Build history of the part. All positions in model axes, mm. A direction names the side the tool comes from. Round coordinates to 2 decimals unless told otherwise and drop trailing zeros. Write each loop counter-clockwise with the first axis right and the second up, starting at its lowest first coordinate (ties: lowest second). Pieces come first, ordered by that corner, then holes. Notation, with made-up numbers: M 50.25,82 L 94.25,82 A23 ccw 94.25,110 Z; hole C -37.5,52 d10. An arc over 180 degrees is marked long. One line per item, written item: value. Start each with the question number.
```python
from build123d import *

# Parameters (mm, degrees)
SKETCH1_W                    = 27.5
SKETCH1_H                    = 23.2
BOSS_EXTRUDE1_REACH          = 62.5
SKETCH2_W                    = 13
SKETCH2_H                    = 10
BOSS_EXTRUDE2_DEPTH          = 16.55326241
BOSS_EXTRUDE3_DEPTH          = 1.5
BOSS_EXTRUDE4_DEPTH          = 1.5
CUT_EXTRUDE1_DEPTH           = 25.05326251
CUT_EXTRUDE2_DEPTH           = 2.5
SKETCH8_R                    = 5.5
BOSS_EXTRUDE5_DEPTH          = 2
SKETCH9_R                    = 2
BOSS_EXTRUDE6_DEPTH          = 8.8
SKETCH10_W                   = 8.8
SKETCH10_H                   = 6
BOSS_EXTRUDE7_DEPTH          = 4.22
CUT_EXTRUDE3_START           = -1
SKETCH11_W                   = 6.8
SKETCH11_H                   = 2.22
CUT_EXTRUDE3_DEPTH           = 5
SKETCH12_R                   = 19.15
BOSS_EXTRUDE8_DEPTH          = 1.5
BOSS_EXTRUDE8_TAPER          = 45
F_7_0_7_DIAMETER_HOLE1_D     = 7
F_7_0_7_DIAMETER_HOLE1_DEPTH = 1.5
SKETCH15_W                   = 1.95
SKETCH15_H                   = 0.1
SKETCH16_W                   = 1.95
SKETCH16_H                   = 0.1
SKETCH17_W                   = 1.95
SKETCH17_H                   = 0.1
SKETCH18_W                   = 1.95
SKETCH18_H                   = 0.1
SKETCH19_W                   = 1.95
SKETCH19_H                   = 0.1
SKETCH20_W                   = 1.95
SKETCH20_H                   = 0.1
SKETCH21_W                   = 2
SKETCH21_H                   = 7
SKETCH22_W                   = 1.95
SKETCH22_H                   = 0.9
SKETCH23_W                   = 1.95
SKETCH23_H                   = 0.9
SKETCH24_W                   = 1.95
SKETCH24_H                   = 0.9
SKETCH25_W                   = 1.95
SKETCH25_H                   = 0.9
SKETCH26_W                   = 1.95
SKETCH26_H                   = 0.9
SKETCH27_W                   = 1.95
SKETCH27_H                   = 0.9


with BuildPart() as part:
    # Sketch1 → Revolve1 (revolve)
    with BuildSketch(Plane.XZ.offset(-27.5)):
        with Locations((41.25, 11.6)):
            Rectangle(SKETCH1_W, SKETCH1_H)
    revolve(axis=Axis((27.5, 27.5, 23.2), (0, 0, -1)))

    # Sketch2 → Boss-Extrude1 (add, up to next)
    with BuildSketch(Plane(origin=(0, 60.5, 0), x_dir=(1, 0, 0), z_dir=(0, 1, 0)), mode=Mode.PRIVATE) as boss_extrude1_sk1:
        with Locations((27.5, -10.7)):
            Rectangle(SKETCH2_W, SKETCH2_H)
    boss_extrude1_tool1 = extrude(boss_extrude1_sk1.sketch, amount=-BOSS_EXTRUDE1_REACH, mode=Mode.PRIVATE) - part.part
    add(boss_extrude1_tool1.solids().sort_by_distance((27.5, 60.5, 10.7))[0])

    # Sketch3 → Boss-Extrude2 (add)
    with BuildSketch(Plane.XY.offset(15.7)):
        with BuildLine():
            Line((34, 60.5), (34, 58))
            add(Edge.make_bspline(
                [(21, 58), (34, 58)],
                knots=[0, 0, 1, 1], degree=1))
            Line((21, 58), (21, 60.5))
            Line((21, 60.5), (34, 60.5))
        make_face()
    extrude(amount=-BOSS_EXTRUDE2_DEPTH)

    # Sketch4 → Boss-Extrude3 (add)
    with BuildSketch(Plane.XY.offset(23.2)):
        with BuildLine():
            Line((64, 32.25), (54.586666462, 32.25))
            ThreePointArc((54.586666462, 32.25), (53.216477037, 17.757679496), (44.640410959, 5.995202578))
            Line((44.640410959, 5.995202578), (66.960616438, 23.785534991))
            ThreePointArc((66.960616438, 23.785534991), (68.483648559, 29.068246028), (64, 32.25))
        make_face()
    extrude(amount=-BOSS_EXTRUDE3_DEPTH)

    # Sketch5 → Boss-Extrude4 (add)
    with BuildSketch(Plane.XY.offset(23.2)):
        with BuildLine():
            Line((-11.960616438, 23.785534991), (10.359589041, 5.995202578))
            ThreePointArc((10.359589041, 5.995202578), (1.783522963, 17.757679496), (0.413333538, 32.25))
            Line((0.413333538, 32.25), (-9, 32.25))
            ThreePointArc((-9, 32.25), (-13.483648559, 29.068246028), (-11.960616438, 23.785534991))
        make_face()
    extrude(amount=-BOSS_EXTRUDE4_DEPTH)

    # Sketch6 → Cut-Extrude1 (cut, through all)
    with BuildSketch(Plane.XY.offset(23.2)):
        with BuildLine():
            Line((63, 25.25), (64, 25.25))
            ThreePointArc((64, 25.25), (66.25, 27.5), (64, 29.75))
            Line((64, 29.75), (63, 29.75))
            ThreePointArc((63, 29.75), (60.75, 27.5), (63, 25.25))
        make_face()
    extrude(amount=-CUT_EXTRUDE1_DEPTH, mode=Mode.SUBTRACT)

    # Sketch7 → Cut-Extrude2 (cut, through all)
    with BuildSketch(Plane(origin=(0, 0, 21.7), x_dir=(-1, 0, 0), z_dir=(0, 0, -1))):
        with BuildLine():
            Line((8, 25.25), (9, 25.25))
            ThreePointArc((9, 25.25), (11.25, 27.5), (9, 29.75))
            Line((9, 29.75), (8, 29.75))
            ThreePointArc((8, 29.75), (5.75, 27.5), (8, 25.25))
        make_face()
    extrude(amount=-CUT_EXTRUDE2_DEPTH, mode=Mode.SUBTRACT)

    # Sketch8 → Boss-Extrude5 (add)
    with BuildSketch(Plane.XY.offset(23.2)):
        with Locations((27.5, 27.5)):
            Circle(SKETCH8_R)
    extrude(amount=BOSS_EXTRUDE5_DEPTH)

    # Sketch9 → Boss-Extrude6 (add)
    with BuildSketch(Plane.XY.offset(25.2)):
        with Locations((27.5, 27.5)):
            Circle(SKETCH9_R)
    extrude(amount=BOSS_EXTRUDE6_DEPTH)

    # Sketch10 → Boss-Extrude7 (add)
    with BuildSketch(Plane(origin=(0, 60.5, 0), x_dir=(-1, 0, 0), z_dir=(0, 1, 0))):
        with Locations((-27.6, 3.14673759)):
            Rectangle(SKETCH10_W, SKETCH10_H)
    extrude(amount=BOSS_EXTRUDE7_DEPTH)

    # Sketch11 → Cut-Extrude3 (cut)
    with BuildSketch(Plane.XY.offset(6.14673759).offset(CUT_EXTRUDE3_START)):
        with Locations((27.6, 62.61)):
            Rectangle(SKETCH11_W, SKETCH11_H)
    extrude(amount=-CUT_EXTRUDE3_DEPTH, mode=Mode.SUBTRACT)

    # Sketch12 → Boss-Extrude8 (add)
    with BuildSketch(Plane(origin=(0, 0, 0), x_dir=(-1, 0, 0), z_dir=(0, 0, -1))):
        with Locations((-27.5, 27.5)):
            Circle(SKETCH12_R)
    extrude(amount=BOSS_EXTRUDE8_DEPTH, taper=BOSS_EXTRUDE8_TAPER)

    # Ø7.0 (7) Diameter Hole1
    with Locations(Plane(origin=(0, 0, -1.5), x_dir=(-1, 0, 0), z_dir=(0, 0, -1))):
        with Locations((-27.5, 27.5)):
            Hole(F_7_0_7_DIAMETER_HOLE1_D / 2, depth=F_7_0_7_DIAMETER_HOLE1_DEPTH)

    # Sketch15 → Cut-Revolve1 (revolve, cut)
    with BuildSketch(Plane(origin=(0, 16.25, 0), x_dir=(1, 0, 0), z_dir=(0, 1, 0))):
        with Locations((8.989428415, -23.15)):
            Rectangle(SKETCH15_W, SKETCH15_H)
    revolve(axis=Axis((8.014428415, 16.25, 23.1), (0, 0, 1)), mode=Mode.SUBTRACT)

    # Sketch16 → Cut-Revolve2 (revolve, cut)
    with BuildSketch(Plane(origin=(0, 5, 0), x_dir=(1, 0, 0), z_dir=(0, 1, 0))):
        with Locations((28.475, -23.15)):
            Rectangle(SKETCH16_W, SKETCH16_H)
    revolve(axis=Axis((27.5, 5, 23.1), (0, 0, 1)), mode=Mode.SUBTRACT)

    # Sketch17 → Cut-Revolve3 (revolve, cut)
    with BuildSketch(Plane(origin=(0, 16.25, 0), x_dir=(1, 0, 0), z_dir=(0, 1, 0))):
        with Locations((47.960571585, -23.15)):
            Rectangle(SKETCH17_W, SKETCH17_H)
    revolve(axis=Axis((46.985571585, 16.25, 23.1), (0, 0, 1)), mode=Mode.SUBTRACT)

    # Sketch18 → Cut-Revolve4 (revolve, cut)
    with BuildSketch(Plane(origin=(0, 38.75, 0), x_dir=(1, 0, 0), z_dir=(0, 1, 0))):
        with Locations((47.960571585, -23.15)):
            Rectangle(SKETCH18_W, SKETCH18_H)
    revolve(axis=Axis((46.985571585, 38.75, 23.1), (0, 0, 1)), mode=Mode.SUBTRACT)

    # Sketch19 → Cut-Revolve5 (revolve, cut)
    with BuildSketch(Plane(origin=(0, 50, 0), x_dir=(1, 0, 0), z_dir=(0, 1, 0))):
        with Locations((28.475, -23.15)):
            Rectangle(SKETCH19_W, SKETCH19_H)
    revolve(axis=Axis((27.5, 50, 23.1), (0, 0, 1)), mode=Mode.SUBTRACT)

    # Sketch20 → Cut-Revolve6 (revolve, cut)
    with BuildSketch(Plane(origin=(0, 38.75, 0), x_dir=(1, 0, 0), z_dir=(0, 1, 0))):
        with Locations((8.989428415, -23.15)):
            Rectangle(SKETCH20_W, SKETCH20_H)
    revolve(axis=Axis((8.014428415, 38.75, 23.1), (0, 0, 1)), mode=Mode.SUBTRACT)

    # Sketch21 → Revolve2 (revolve)
    with BuildSketch(Plane(origin=(0, 27.5, 0), x_dir=(1, 0, 0), z_dir=(0, 1, 0))):
        with Locations((28.5, 3.5)):
            Rectangle(SKETCH21_W, SKETCH21_H)
    revolve(axis=Axis((27.5, 27.5, -7), (0, 0, 1)))

    # Sketch22 → Revolve3 (revolve)
    with BuildSketch(Plane(origin=(0, 16.25, 0), x_dir=(1, 0, 0), z_dir=(0, 1, 0))):
        with Locations((47.960571585, 0.45)):
            Rectangle(SKETCH22_W, SKETCH22_H)
    revolve(axis=Axis((46.985571585, 16.25, -0.9), (0, 0, 1)))

    # Sketch23 → Revolve4 (revolve)
    with BuildSketch(Plane(origin=(0, 5, 0), x_dir=(1, 0, 0), z_dir=(0, 1, 0))):
        with Locations((28.475, 0.45)):
            Rectangle(SKETCH23_W, SKETCH23_H)
    revolve(axis=Axis((27.5, 5, -0.9), (0, 0, 1)))

    # Sketch24 → Revolve5 (revolve)
    with BuildSketch(Plane(origin=(0, 16.25, 0), x_dir=(1, 0, 0), z_dir=(0, 1, 0))):
        with Locations((8.989428415, 0.45)):
            Rectangle(SKETCH24_W, SKETCH24_H)
    revolve(axis=Axis((8.014428415, 16.25, -0.9), (0, 0, 1)))

    # Sketch25 → Revolve6 (revolve)
    with BuildSketch(Plane(origin=(0, 38.75, 0), x_dir=(1, 0, 0), z_dir=(0, 1, 0))):
        with Locations((8.989428415, 0.45)):
            Rectangle(SKETCH25_W, SKETCH25_H)
    revolve(axis=Axis((8.014428415, 38.75, -0.9), (0, 0, 1)))

    # Sketch26 → Revolve7 (revolve)
    with BuildSketch(Plane(origin=(0, 50, 0), x_dir=(1, 0, 0), z_dir=(0, 1, 0))):
        with Locations((28.475, 0.45)):
            Rectangle(SKETCH26_W, SKETCH26_H)
    revolve(axis=Axis((27.5, 50, -0.9), (0, 0, 1)))

    # Sketch27 → Revolve8 (revolve)
    with BuildSketch(Plane(origin=(0, 38.75, 0), x_dir=(1, 0, 0), z_dir=(0, 1, 0))):
        with Locations((47.960571585, 0.45)):
            Rectangle(SKETCH27_W, SKETCH27_H)
    revolve(axis=Axis((46.985571585, 38.75, -0.9), (0, 0, 1)))


solid = part.part
```
Item 1: Cut at B-B, the plane x = 62. Write the cut outline in (y, z), plus the area to 3 significant figures.
Item 2: Two-plate mould, pull along Y, no slides. Class faces 5 (the cylindrical face through (60.75, 27.55, 22.46)), 6 (the flat face through (28, 59, -0.853)), 7 (the cylindrical face through (28.423, 25.726, 29.538)): pulls with the +Y half, pulls with the -Y half, needs draft (parallel to the pull), parting line crosses it, or undercut.
Item 3: Cut at A-A, the plane z = 4. Count the separate pieces of the cut face and the enclosed holes in it, plus the area to 3 significant figures.
Item 4: Cut at D-D, the plane z = 28.5. Write the cut outline in (x, y), plus the area to 3 significant figures.
Item 5: Drop flat-ended pins along their axis: pin 1 (3 mm diameter, centred on y = 58, z = 5, fed in from +X); pin 2 (6 mm diameter, centred on x = 27.5, y = 50, fed in from -Z); pin 3 (2 mm diameter, centred on x = 28.5, y = 6, fed in from +Z). Give the stop position or say it passes through.
Item 6: Cut at C-C, the plane y = 5. Write the cut outline in (x, z).
Item 7: Drill centre lines: line 1 (Y direction, x = 27.5, z = -0.7); line 2 (Z direction, x = 15, y = 35); line 3 (Z direction, x = 58, y = 27.5). Where is each one in solid material? Low to high.
Item 8: Which spindle directions (+Z, -Z, +X, -X, +Y, -Y) get a long thin tool onto all of the face, cutting with end or side? Do faces 1 (the flat face through (8, 39, -0.9)), 2 (the flat face through (-0.957, 15.015, 22.46)), 3 (the flat face through (31, 63, 3)), 4 (the flat face through (47, 16, 23.1)). Say none if no direction does.
Computed values:
1. outline: M 19.83,21.7 L 25.48,21.7 L 25.48,23.2 L 19.83,23.2 Z; M 29.52,21.7 L 32.25,21.7 L 32.25,23.2 L 29.52,23.2 Z
1. area: 12.6 mm2
2. face 5: undercut
2. face 6: needs draft
2. face 7: parting line crosses it
3. separate pieces: 2
3. enclosed holes: 1
3. area: 2,430 mm2
4. outline: C 27.5,27.5 d4
4. area: 12.6 mm2
5. pin 1: stops at x = 34
5. pin 2: stops at z = -0.9
5. pin 3: stops at z = 23.2
6. outline: M 11.69,0 L 25.55,0 L 25.55,-0.9 L 29.45,-0.9 L 29.45,0 L 43.31,0 L 43.31,23.2 L 29.45,23.2 L 29.45,23.1 L 25.55,23.1 L 25.55,23.2 L 11.69,23.2 Z
7. line 1: y = 3.05 to 6.95, 9.05 to 24, 25.5 to 29.5, 31 to 45.95, 48.05 to 51.95, 58 to 60.5
7. line 2: z = -1.5 to 23.2
7. line 3: z = 21.7 to 23.2
8. face 1: -Z, -X, +Y
8. face 2: +Z, -Z, -X, -Y
8. face 3: -Z
8. face 4: +Z
